Part print with two shaded views. Sizes in mm from the minimum x, y, z corner. Round coordinates to 2 decimals unless told otherwise and drop trailing zeros. Loops run counter-clockwise (first coordinate to the right, second up) from the corner with the lowest first, then second, coordinate; pieces in that order, holes last.
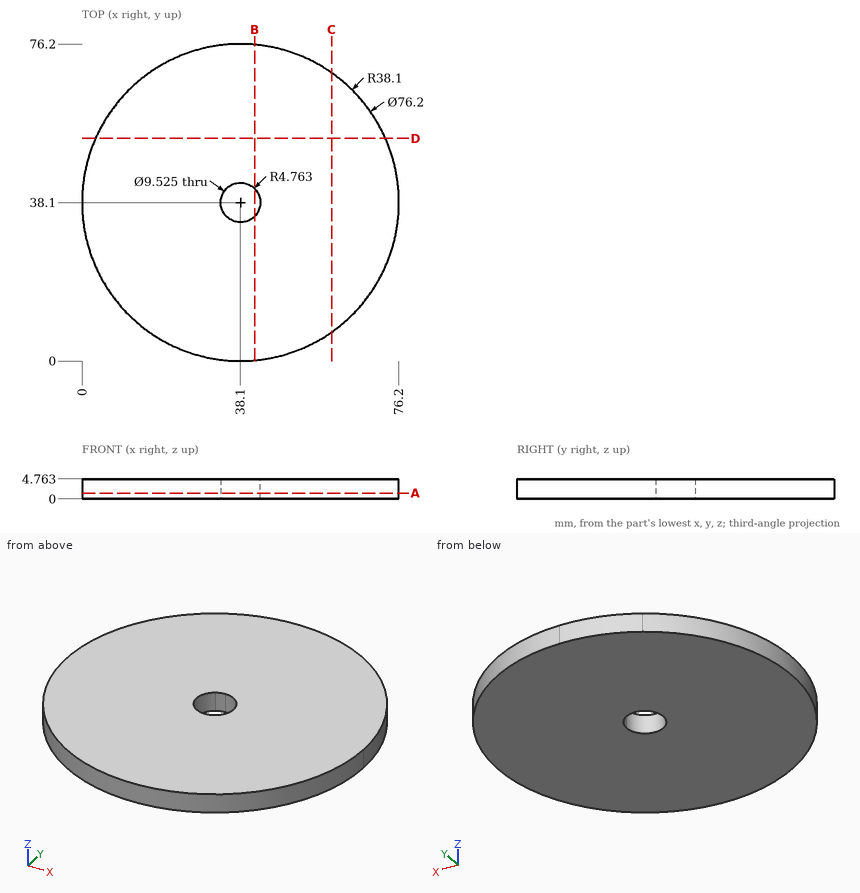
Item 1: Cut at C-C (x = 60). List the corners of the cut face in (y, z).
Verdict:
outline: (6.92, 0) - (69.28, 0) - (69.28, 4.76) - (6.92, 4.76) - close
Item 2: Cut at A-A (z = 1.35). List the corners of the cut face in (x, y) (1 decimal).
Verdict:
outline: circle Ø76.2 at (38.1, 38.1); hole circle Ø9.5 at (38.1, 38.1)
Item 3: Cut at B-B (x = 41.5). List the corners of the cut face in (y, z) (1 decimal).
Verdict:
outline: (0.2, 0) - (34.8, 0) - (34.8, 4.8) - (0.2, 4.8) - close; (41.4, 0) - (76, 0) - (76, 4.8) - (41.4, 4.8) - close
Item 4: Cut at D-D (y = 53.5). List the corners of the cut face in (x, z), plus the area to 3 significant figures.
Verdict:
outline: (3.25, 0) - (72.95, 0) - (72.95, 4.76) - (3.25, 4.76) - close
area: 332 mm2
Item 5: Wall check: L1, parallel to Y at x = 38.1, z = 3.75; L2, parallel to X at y = 37, z = 3.35 (1 decimal); L3, parallel to Y at x = 33, z = 1.85. Give the ranges that are in metal, low to high.
Verdict:
L1: y = 0 to 33.34, 42.86 to 76.2
L2: x = 0 to 33.5, 42.7 to 76.2
L3: y = 0.34 to 75.86
Item 6: Flat gauge pin, fed straight in: P1, Ø1, axis at x = 32, z = 3.5, coming from the -Y side. Where does the tip first touch, or does it go through?
Verdict:
P1: stops at y = 0.41
